from build123d import *

# Parameters (mm, degrees)
BOSS_EXTRUDE1_DEPTH = 12.7
SKETCH2_R           = 2.5
CUT_EXTRUDE1_DEPTH  = 16.24
SKETCH3_W           = 7.62
SKETCH3_H           = 3.81
CUT_EXTRUDE2_DEPTH  = 83.6200001


with BuildPart() as part:
    # Sketch1 → Boss-Extrude1 (new body)
    with BuildSketch(Plane.XY):
        with BuildLine():
            Line((-41.31, 0), (41.31, 0))
            Line((41.31, 0), (41.31, -15.24))
            ThreePointArc((41.31, -15.24), (0, -11.677615661), (-41.31, -15.24))
            Line((-41.31, -15.24), (-41.31, 0))
        make_face()
    extrude(amount=BOSS_EXTRUDE1_DEPTH)

    # Sketch2 → Cut-Extrude1 (cut, through all)
    with BuildSketch(Plane(origin=(0, 0, 0), x_dir=(1, 0, 0), z_dir=(0, 1, 0))):
        with Locations((-34.31, -6.35)):
            Circle(SKETCH2_R)
        with Locations((34.31, -6.35)):
            Circle(SKETCH2_R)
    extrude(amount=-CUT_EXTRUDE1_DEPTH, mode=Mode.SUBTRACT)

    # Sketch3 → Cut-Extrude2 (cut, through all)
    with BuildSketch(Plane(origin=(41.31, 0, 0), x_dir=(0, 0, -1), z_dir=(1, 0, 0))):
        with Locations((-6.35, -13.335)):
            Rectangle(SKETCH3_W, SKETCH3_H)
    extrude(amount=-CUT_EXTRUDE2_DEPTH, mode=Mode.SUBTRACT)


solid = part.part
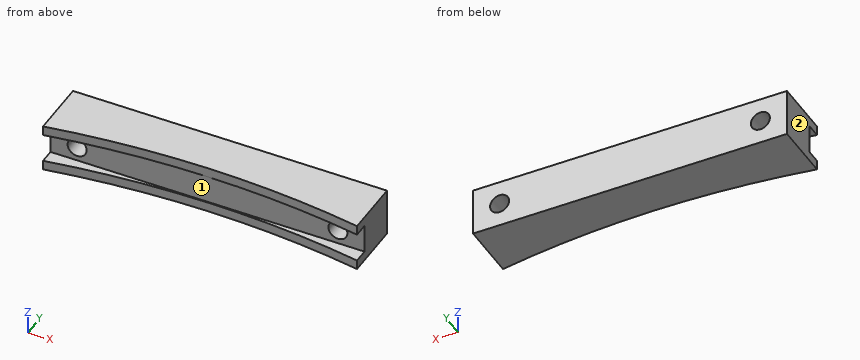
Could you check a few things on this model? Use its own coordinates, in mm. Face numbers are marked on the shaded views. A direction names the side the tool comes from. Coordinates: 2 decimals unless noted, no trailing zeros. Order: outer loops, then holes, each group sorted by start corner. A loop starts at its lowest first (then second) coordinate and runs counter-clockwise, first axis right, second up. Notation, with made-up numbers: (67, 23) -> (85, 23) arc R24 ccw to (85, 43) -> close; hole circle Ø6 at (-36.75, 30.25). An arc over 180 degrees is marked (long way). One line per item, written item: value. Start each with the question number.
1) Imagine slicing it at D-D on y = -13.75. List the corners of the cut face in (x, z) for me.
2) Imagine slicing it at A-A on z = 6.35. List the corners of the cut face in (x, y) for me, plus the area to 3 significant figures.
3) Imagine slicing it at C-C on x = 34.31. List the corners of the cut face in (y, z) for me, plus the area to 3 significant figures.
4) If I drill on L1, parallel to X at y = -4, z = 6.35; L2, parallel to X at y = -2.5, z = 5.25 (3 decimals); L3, parallel to Z at x = -34.31, y = -7, over which ranges is the centre line in solid material (lowest first)? Write a range as [from, to].
5) I'm going to push flat-ended pins straight in: pin 1 (2 mm diameter, centred on x = -28.5, z = 3.5, fed in from +Y); pin 2 (4.5 mm diameter, centred on x = -34.31, z = 6.35, fed in from -Y); pin 3 (4 mm diameter, centred on x = 1.5, z = 7.5, fed in from -Y). Where does each tip first touch, or does it pass through?
6) Imagine slicing it at B-B on y = -3.25. List the corners of the cut face in (x, z) for me.
7) Which directions (+Z, -Z, +X, -X, +Y, -Y) give clear straight access to the entire face, cutting with the end or side of a thin tool? Please do the marked faces 1 and 2.
Answer list:
1. outline: (-41.31, 0) -> (-31.56, 0) -> (-31.56, 2.54) -> (-41.31, 2.54) -> close; (-41.31, 10.16) -> (-31.56, 10.16) -> (-31.56, 12.7) -> (-41.31, 12.7) -> close; (31.56, 0) -> (41.31, 0) -> (41.31, 2.54) -> (31.56, 2.54) -> close; (31.56, 10.16) -> (41.31, 10.16) -> (41.31, 12.7) -> (31.56, 12.7) -> close
2. outline: (-41.31, -11.43) -> (-36.81, -11.43) -> (-36.81, 0) -> (-41.31, 0) -> close; (-31.81, -11.43) -> (31.81, -11.43) -> (31.81, 0) -> (-31.81, 0) -> close; (36.81, -11.43) -> (41.31, -11.43) -> (41.31, 0) -> (36.81, 0) -> close
2. area: 830 mm2
3. outline: (-14.13, 0) -> (0, 0) -> (0, 3.85) -> (-11.43, 3.85) -> (-11.43, 2.54) -> (-14.13, 2.54) -> close; (-14.13, 10.16) -> (-11.43, 10.16) -> (-11.43, 8.85) -> (0, 8.85) -> (0, 12.7) -> (-14.13, 12.7) -> close
3. area: 102 mm2
4. L1: x = [-41.31, -36.81], [-31.81, 31.81], [36.81, 41.31]
4. L2: x = [-41.31, -36.555], [-32.065, 32.065], [36.555, 41.31]
4. L3: z = [0, 3.85], [8.85, 12.7]
5. pin 1: stops at y = 0
5. pin 2: passes through
5. pin 3: stops at y = -11.43
6. outline: (-41.31, 0) -> (41.31, 0) -> (41.31, 12.7) -> (-41.31, 12.7) -> close; hole circle Ø5 at (-34.31, 6.35); hole circle Ø5 at (34.31, 6.35)
7. face 1: +X, -X, -Y
7. face 2: +Z, -Z, -X, +Y, -Y
